Geometry check sheet. Reference: the model listing, model coordinates, mm. Face numbers are marked on the shaded views. Give positions to 0.01 mm unless a question says otherwise; leave off trailing zeros. Write item = value, one per line. Start each with the question number.
(1) Draft check along Y on the marked faces 1, 2 and 3. Enter one of: pulls with the +Y half, pulls with the -Y half, needs draft (parallel to the pull), parting line crosses it, or undercut.
(2) Thickness scan on L1, parallel to X at y = -27, z = 0 (3 decimals); L2, parallel to Z at x = -57, y = -31; L3, parallel to Z at x = 65, y = -18. Record the ranges inside material, lowest first.
(3) Depth check by flat-ended pin: pin 1 Ø1 at (x, y) = (55, -13.5) entering from +Z; pin 2 Ø5 at (x, z) = (0, 0) entering from -Y; pin 3 Ø2 at (x, y) = (15, -20) entering from -Z; pin 4 Ø4 at (x, z) = (-41.5, -65.5) entering from +Y. Enter the tip coordinate at first touch or a pass-through.
```python
from build123d import *

# Parameters (mm, degrees)
F2_R    = 0.508
F3_SIZE = 1.524


with BuildPart() as f1:
    # F0 (on Right) → F1 (revolve)
    with BuildSketch(Plane.YZ):
        Polygon((-21.1680062206, 0), (0, 0), (0, 79.00924), (-14.6116351058, 79.00924), (-15.3736351058, 78.24724), (-15.875, 78.24724), (-15.875, 79.00924), (-15.875, 85.09), (-34.925, 85.09), (-34.925, 6.35), (-29.425738686, 3.175), (-23.075738686, 3.175), align=None)
    revolve(axis=Axis((0, -21.1680062206, 0), (0, 1, 0)))

    # F2
    f2_edges = [f1.edges().sort_by_distance(p)[0] for p in [
        (0, -15.875, -85.09),
    ]]
    fillet(f2_edges, radius=F2_R)

    # F3
    f3_edges = [f1.edges().sort_by_distance(p)[0] for p in [
        (0, 0, -79.00924),
        (0, -34.925, -85.09),
    ]]
    chamfer(f3_edges, length=F3_SIZE)


solid = f1.part
```
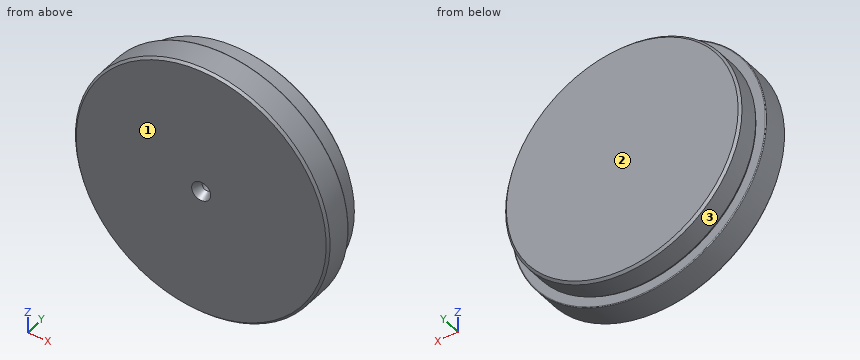
Model answer:
q1.face_1 = pulls with the -Y half
q1.face_2 = pulls with the +Y half
q1.face_3 = needs draft
q2.L1 = -85.09 to -3.175, 3.175 to 85.09
q2.L2 = -63.18 to 63.18
q2.L3 = -54.91 to 54.91
q3.pin_1 = 57.2
q3.pin_2 = -22.67
q3.pin_3 = -83.93
q3.pin_4 = 0
